Geometry check sheet. Reference: drawing and pictorial views, mm from the part's lowest x, y, z. A direction names the side the tool comes from. Give positions to 0.01 mm unless a question says otherwise; leave off trailing zeros. Loops run counter-clockwise (first coordinate to the right, second up) from the corner with the lowest first, then second, coordinate; pieces in that order, holes last. Notation, with made-up numbers: (75, -25.75) - (86, -25.75) arc R21 cw to (86, -6.75) - close; hole circle Ø9 at (82.5, -27). An arc over 180 degrees is marked (long way). Answer in a Markdown table with one row per item. Add a question column.
(1) Thickness scan on L1, parallel to X at y = 8.75, z = 0.65; L2, parallel to Z at x = 4.25, y = 26.75; L3, parallel to Y at x = 8.75, z = 0.8. Record the ranges inside material, lowest first.
(2) Set-up check for the marked faces 5 and 6: record each of +Z, -Z, +X, -X, +Y, -Y from which the full face is reachable in a straight line by a thin tool's end or side.
(3) Go/stop test with flat-tipped pins: P1, Ø4, axis at x = 14.5, y = 9, coming from the +Z side; P2, Ø0.8, axis at x = 16, z = 2, coming from the +Y side; P3, Ø2, axis at y = 17, z = 3, coming from the +X side. Record where each tip stops, or that it passes through.
(4) Sectioned sample at A-A on z = 1.5. Enter the section's corners in (x, y).
(5) Sectioned sample at C-C on x = 1.75. Enter the section's corners in (y, z).
(6) Sectioned sample at B-B on y = 14.75. Enter the section's corners in (x, z), then the cut area to 3 significant figures.
(7) Draft check along X on the marked faces 1, 2, 3 and 4. Enter one of: released by +X, released by -X, zero draft, split by the parting line, or undercut.
(8) Sectioned sample at D-D on x = 8.5. Enter the section's corners in (y, z), then the cut area to 3 significant figures.
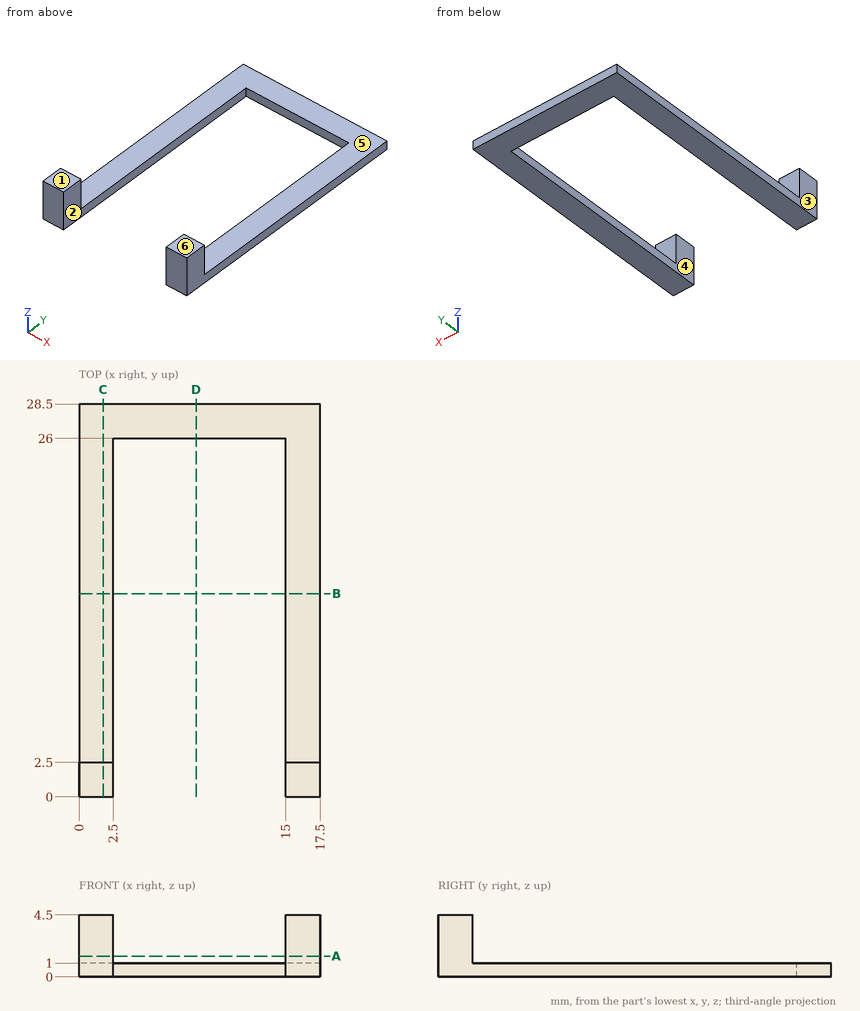
Reply:
| question | item | result |
|---|---|---|
| 1 | L1 | 0 to 2.5, 15 to 17.5 |
| 1 | L2 | 0 to 1 |
| 1 | L3 | 26 to 28.5 |
| 2 | face 5 | +Z, +X, -X, +Y |
| 2 | face 6 | +Z, +X, -X, +Y, -Y |
| 3 | P1 | z = 1 |
| 3 | P2 | y = 2.5 |
| 3 | P3 | through |
| 4 | outline | (0, 0) - (2.5, 0) - (2.5, 2.5) - (0, 2.5) - close; (15, 0) - (17.5, 0) - (17.5, 2.5) - (15, 2.5) - close |
| 5 | outline | (0, 0) - (28.5, 0) - (28.5, 1) - (2.5, 1) - (2.5, 4.5) - (0, 4.5) - close |
| 6 | outline | (0, 0) - (2.5, 0) - (2.5, 1) - (0, 1) - close; (15, 0) - (17.5, 0) - (17.5, 1) - (15, 1) - close |
| 6 | area | 5.00 mm^2 |
| 7 | face 1 | zero draft |
| 7 | face 2 | undercut |
| 7 | face 3 | released by -X |
| 7 | face 4 | undercut |
| 8 | outline | (26, 0) - (28.5, 0) - (28.5, 1) - (26, 1) - close |
| 8 | area | 2.50 mm^2 |
